Geometry check sheet. Reference: the model listing, model coordinates, mm. Face numbers are marked on the shaded views. A direction names the side the tool comes from. Round coordinates to 2 decimals unless told otherwise and drop trailing zeros. Write each loop counter-clockwise with the first axis right and the second up, starting at its lowest first coordinate (ties: lowest second). Pieces come first, ordered by that corner, then holes. Notation, with made-up numbers: M 12.25,-25.75 L 45.25,-25.75 A18 ccw 45.25,-3.75 Z; hole C -2.5,53.5 d7. An arc over 180 degrees is marked long. Put each result on its own line as item: value. Start each with the question number.
(1) Section check A-A on z = 6. Record the cut outline in (x, y).
(2) Material ranges on probe 1 along Z at (x, y) = (4.25, -0.5); probe 2 along X at (y, z) = (-1.2, 7.75); probe 3 along Y at (x, z) = (14.5, 3.5), recorded low to high.
(3) Section check C-C on y = -0.8. Record the cut outline in (x, z).
(4) Section check B-B on x = 15. Record the cut outline in (y, z), then the cut area to 3 significant figures.
(5) Gauge pin test, flat ends, axial feed: pin 1 (4 mm diameter, centred on x = 6.5, z = 2.5, fed in from -Y); pin 2 (2 mm diameter, centred on x = 7, z = 6, fed in from -Y). Record the tip position at first contact, or that the pin passes through.
(6) Mould release check, pull along X, two halves, no side actions. Record for the marked faces 4, 5 and 6: pulls with the +X half, pulls with the -X half, needs draft (parallel to the pull), parting line crosses it, or undercut.
(7) Section check D-D on z = 1.75. Record the cut outline in (x, y), then the cut area to 3 significant figures.
(8) Tool access check on the marked faces 1, 2 and 3. Record the directions out of +Z, -Z, +X, -X, +Y, -Y that give a thin tool (end or side, any length) a straight path to the whole face; none if there is none.
Autodesk Fusion 360 part; units mm, degrees
sketch "Sketch1" plane through (0, 0, 0) normal (0, 1, 0) x (1, 0, 0)
  line L0 (0, 0) -> (16, 0)
  line L1 (16, -10) -> (0, -10)
  line L2 (0, -10) -> (0, 0)
  line L3 (1.5, -8.5) -> (14.5, -8.5)
  line L4 (14.5, -1.5) -> (1.5, -1.5)
  line L5 (1.5, -1.5) -> (1.5, -8.5)
  line L6 (14.5, -7.5) -> (16, -7.5)
  line L7 (16, -2.5) -> (14.5, -2.5)
  line L8 (16, 0) -> (16, -2.5)
  line L9 (16, -7.5) -> (16, -10)
  line L10 (14.5, -8.5) -> (14.5, -7.5)
  line L11 (14.5, -2.5) -> (14.5, -1.5)
  line L12 (0, -10) -> (16, -10)
  line L13 (16, -10) -> (16, 0)
  line L14 (16, 0) -> (0, 0)
  line L15 (0, 0) -> (0, -10)
  dimension "d2" = 1.5
  dimension "d3" = 1.5
  dimension "d4" = 1.5
  dimension "d5" = 1.5
  dimension "d7" = 1
  dimension "d8" = 1
  dimension "d9" = 13
  dimension "d10" = 10
extrude "Extrude1" add sketch "Sketch1" along normal blind 1
extrude "Extrude2" add sketch "Sketch1" against normal blind 1.6 contours L0 L1 L2 L3 L4 L5 L6 L7 L8 L9 L10 L11 L12 L13 L14 L15
fillet "Fillet1" radius 0.5 8 edges at (8, 1, 10) (0, 1, 5) (8, 1, 0) (16, 1, 5) (16, -0.3, 0) (0, -0.3, 0) (0, -0.3, 10) (16, -0.3, 10)
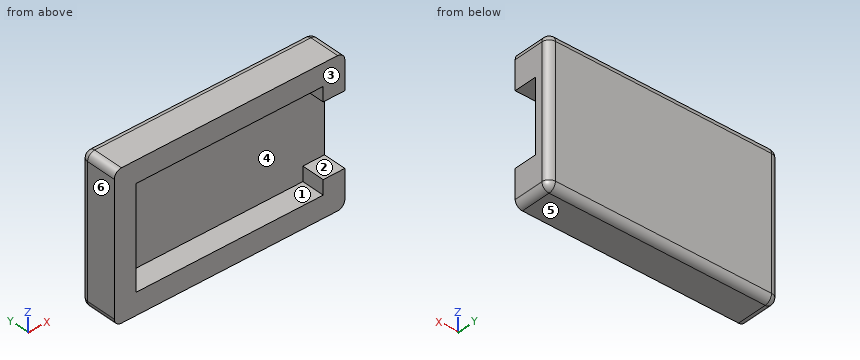
Answers follow:
1. outline: M 0,-1.6 L 1.5,-1.6 L 1.5,0 L 16,0 L 16,0.5 A0.5 ccw 15.5,1 L 0.5,1 A0.5 ccw 0,0.5 Z
2. probe 1: z = 0 to 1.5, 8.5 to 10
2. probe 2: x = 0 to 1.5, 14.5 to 16
2. probe 3: y = 0 to 1
3. outline: M 0,0.5 A0.5 ccw 0.5,0 L 15.5,0 A0.5 ccw 16,0.5 L 16,2.5 L 14.5,2.5 L 14.5,1.5 L 1.5,1.5 L 1.5,8.5 L 14.5,8.5 L 14.5,7.5 L 16,7.5 L 16,9.5 A0.5 ccw 15.5,10 L 0.5,10 A0.5 ccw 0,9.5 Z
4. outline: M -1.6,0 L 0.5,0 A0.5 ccw 1,0.5 L 1,9.5 A0.5 ccw 0.5,10 L -1.6,10 L -1.6,7.5 L 0,7.5 L 0,2.5 L -1.6,2.5 Z
4. area: 17.9 mm^2
5. pin 1: stops at y = -1.6
5. pin 2: stops at y = 0
6. face 4: undercut
6. face 5: needs draft
6. face 6: pulls with the -X half
7. outline: M 0,-1.6 L 1.5,-1.6 L 1.5,0 L 14.5,0 L 14.5,-1.6 L 16,-1.6 L 16,0.5 A0.5 ccw 15.5,1 L 0.5,1 A0.5 ccw 0,0.5 Z
7. area: 20.7 mm^2
8. face 1: -Y
8. face 2: +X, -Y
8. face 3: +Z, -Z, +X, -X, -Y
